Read the model definition and answer for the solid it produces. Units are mm, in the model's axes. Face numbers are marked on the shaded views. A direction names the side the tool comes from. Round coordinates to 2 decimals unless told otherwise and drop trailing zeros. Write each loop counter-clockwise with the first axis right and the second up, starting at its lowest first coordinate (ties: lowest second). Pieces come first, ordered by that corner, then holes.
from build123d import *

# Parameters (mm, degrees)
F0_R     = 4.5926712991
F1_DEPTH = 6.35
F2_W     = 2.3739238567
F2_H     = 8.0889270103
F2_W_2   = 2.3739274609
F2_H_2   = 7.4734649694
F2_R     = 1.2680453983
F2_R_2   = 1.2379691671
F3_DEPTH = 3.175


# Not quite as in the source:
# - a length typed as a fraction of an inch, garbled in the dataset ("3 / 203.2 mm" for 3/8 in), is restored


with BuildPart() as f1:
    # F0 (on Top) → F1 (new body)
    with BuildSketch(Plane.XY):
        with BuildLine():
            Line((-63.5, 0), (0, 0))
            Line((0, 0), (0, 25.4))
            Line((0, 25.4), (-22.4021356553, 25.4))
            ThreePointArc((-22.4021356553, 25.4), (-31.3605917618, 34.9369900473), (-40.3190478683, 25.4))
            Line((-40.3190478683, 25.4), (-63.5, 25.4))
            Line((-63.5, 25.4), (-63.5, 0))
        make_face()
        with Locations((-31.3605917618, 25.960986396)):
            Circle(F0_R, mode=Mode.SUBTRACT)
    extrude(amount=F1_DEPTH)

    # F2 (on face) → F3 (cut)
    with BuildSketch(Plane.XY.offset(6.35)):
        with BuildLine():
            Line((-47.8143577063, 14.1739739048), (-45.6251816468, 16.6567004661))
            ThreePointArc((-45.6251816468, 16.6567004661), (-60.5221954701, 12.262678636), (-46.5953443626, 5.3872683266))
            Line((-46.5953443626, 5.3872683266), (-49.6666999843, 7.1012593313))
            ThreePointArc((-49.6666999843, 7.1012593313), (-57.1721052058, 12.8458444774), (-47.8143577063, 14.1739739048))
        make_face()
        Polygon((-20.7504647221, 18.5370575163), (-32.6200858075, 18.5370575163), (-32.6200858075, 15.7841322933), (-27.6963894798, 15.7841322933), (-27.6963894798, 3.8538966697), (-25.0586963057, 3.8538966697), (-25.0586963057, 15.7841322933), (-20.7504647221, 15.7841322933), align=None)
        with BuildLine():
            Line((-8.0016118277, 15.7841322933), (-10.2876118277, 15.7841322933))
            Line((-10.2876118277, 15.7841322933), (-10.2876118277, 3.7659732636))
            Line((-10.2876118277, 3.7659732636), (-8.0016118277, 3.7659732636))
            Line((-8.0016118277, 3.7659732636), (-8.0016118277, 6.1422445658))
            ThreePointArc((-8.0016118277, 6.1422445658), (-7.7348762924, 6.9209360412), (-7.0467135382, 7.3725335205))
            ThreePointArc((-7.0467135382, 7.3725335205), (-6.358550784, 6.9209360412), (-6.0918152487, 6.1422445658))
            Line((-6.0918152487, 6.1422445658), (-6.0918152487, 3.8510074993))
            Line((-6.0918152487, 3.8510074993), (-4.2027005772, 3.8510074993))
            Line((-4.2027005772, 3.8510074993), (-4.2027005772, 8.5050527784))
            ThreePointArc((-4.2027005772, 8.5050527784), (-4.5746749651, 9.4030783905), (-5.4727005772, 9.7750527784))
            Line((-5.4727005772, 9.7750527784), (-6.7316118277, 9.7750527784))
            ThreePointArc((-6.7316118277, 9.7750527784), (-7.6296374398, 10.1470271663), (-8.0016118277, 11.0450527784))
            Line((-8.0016118277, 11.0450527784), (-8.0016118277, 15.7841322933))
        make_face()
        with BuildLine():
            ThreePointArc((-6.7316118277, 7.4122445658), (-6.8904089113, 7.4022776948), (-7.0467135382, 7.3725335205))
            ThreePointArc((-7.0467135382, 7.3725335205), (-7.203018165, 7.4022776948), (-7.3618152487, 7.4122445658))
            Line((-7.3618152487, 7.4122445658), (-6.7316118277, 7.4122445658))
        make_face(mode=Mode.SUBTRACT)
        Polygon((-36.7524705789, 17.2182109293), (-38.9505494254, 17.2182109293), (-38.9505494254, 13.3495927722), (-40.7090139442, 13.3495927722), (-40.7090139442, 11.8549002739), (-38.9505494254, 11.8549002739), (-38.9505494254, 3.7659732636), (-36.7524705789, 3.7659732636), (-36.7524705789, 11.8549002739), (-34.9940096642, 11.8549002739), (-34.9940096642, 13.3495927722), (-36.7524705789, 13.3495927722), align=None)
        with BuildLine():
            Line((-12.6827618144, 8.0606505512), (-11.5731045271, 9.2428652738))
            ThreePointArc((-11.5731045271, 9.2428652738), (-17.6629146287, 7.19801004), (-11.6904523614, 4.8322301544))
            Line((-11.6904523614, 4.8322301544), (-13.1890844097, 5.6123530456))
            ThreePointArc((-13.1890844097, 5.6123530456), (-16.0358025283, 7.4775754374), (-12.6827618144, 8.0606505512))
        make_face()
        with Locations((-43.7423610944, 7.8104367687)):
            Rectangle(F2_W, F2_H)
        with Locations((-19.5635009916, 7.5906291544)):
            Rectangle(F2_W_2, F2_H_2)
        with Locations((-19.4316163329, 13.5254395845)):
            Circle(F2_R)
        with Locations((-43.7423610944, 13.7892089019)):
            Circle(F2_R_2)
        with BuildLine():
            ThreePointArc((-7.3618152487, 7.4122445658), (-7.203018165, 7.4022776948), (-7.0467135382, 7.3725335205))
            ThreePointArc((-7.0467135382, 7.3725335205), (-6.8904089113, 7.4022776948), (-6.7316118277, 7.4122445658))
            Line((-6.7316118277, 7.4122445658), (-7.3618152487, 7.4122445658))
        make_face()
    extrude(amount=-F3_DEPTH, mode=Mode.SUBTRACT)


solid = f1.part
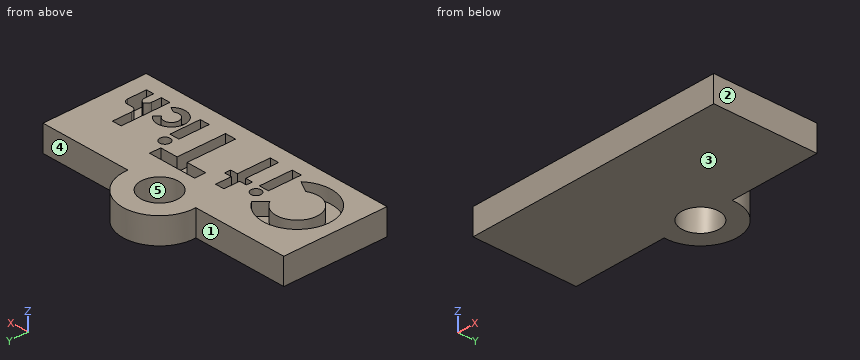
Q1. Section B-B (z = 1.5) is taken. Determine the outline of the cut face in (x, y), then the cut area to 3 significant figures.
Verdict:
outline: (-63.5, 0) - (0, 0) - (0, 25.4) - (-22.4, 25.4) arc R8.98 ccw (long way) to (-40.32, 25.4) - (-63.5, 25.4) - close; hole circle Ø9.19 at (-31.36, 25.96)
area: 1,680 mm2
Q2. Determine the mould class of the marked faces 3, 4 and 5 for opening direction Y: pulls with the +Y half, pulls with the -Y half, needs draft (parallel to the pull), parting line crosses it, or undercut.
Verdict:
face 3: needs draft
face 4: pulls with the +Y half
face 5: undercut
Q3. Straight lines are drawn through the part: probe 1 along Y at (x, z) = (-48.5, 3.5); probe 2 along Y at (x, z) = (-35.5, 5.25); probe 3 along Y at (x, z) = (-40.5, 2.75). For each, find the intervals that lie inside material, in ascending order.
Verdict:
probe 1: y = 0 to 4.08, 6.45 to 15.08, 19.01 to 25.4
probe 2: y = 0 to 11.85, 13.35 to 23.97, 27.95 to 33.93
probe 3: y = 0 to 25.4
Q4. Flat-ended cylindrical pins translate along their axes: pin 1 Ø2.5 at (x, z) = (-23.5, 5.5) entering from +Y; pin 2 Ø1.1 at (x, z) = (-37.5, 5) entering from +Y; pin 3 Ø1.9 at (x, z) = (-36, 4.5) entering from +Y. Find the tip coordinate at first contact, or state that the pin passes through.
Verdict:
pin 1: stops at y = 32.03
pin 2: stops at y = 32.98
pin 3: stops at y = 34.14
Q5. Section A-A (x = -31.5) is taken. Determine the outline of the cut face in (y, z) (3 decimals).
Verdict:
outline: (0, 0) - (21.37, 0) - (21.37, 6.35) - (18.537, 6.35) - (18.537, 3.175) - (15.784, 3.175) - (15.784, 6.35) - (0, 6.35) - close; (30.552, 0) - (34.936, 0) - (34.936, 6.35) - (30.552, 6.35) - close
Q6. Which of the six approach directions +Z, -Z, +X, -X, +Y, -Y give full straight-line access (tool end or side, diameter ignored) to the marked faces 1 and 2?
Verdict:
face 1: +Z, -Z, -X, +Y
face 2: +Z, -Z, +X, +Y, -Y
Q7. Section C-C (x = -56) is taken. Determine the outline of the cut face in (y, z) (3 decimals), then the cut area to 3 significant figures.
Verdict:
outline: (0, 0) - (25.4, 0) - (25.4, 6.35) - (18.977, 6.35) - (18.977, 3.175) - (15.002, 3.175) - (15.002, 6.35) - (8.093, 6.35) - (8.093, 3.175) - (4.118, 3.175) - (4.118, 6.35) - (0, 6.35) - close
area: 136 mm2
Q8. Section D-D (z = 4.75) is taken. State how many separate pieces and enclosed holes the cut face has, then the cut area to 3 significant figures.
Verdict:
separate pieces: 1
enclosed holes: 10
area: 1,370 mm2
